from build123d import *

# Parameters (mm, degrees)
F0_W          = 645
F0_H          = 495
F1_DEPTH      = 82
F3_DEPTH      = 322.501
F3_DEPTH_BACK = 495
F5_DEPTH      = 365
F5_DEPTH_BACK = 341
F6_T          = 18
F6_T3_DEPTH   = 505.2074342574
F6_T5_DEPTH   = 651


# Not quite as in the source:
# - a shell that OpenCascade refuses in one call is made with other operations: the cavity is built on its own and cut out


with BuildPart() as f1:
    # F0 (on Top) → F1 (new body)
    with BuildSketch(Plane.XY):
        Rectangle(F0_W, F0_H)
    extrude(amount=-F1_DEPTH)

    # F2 (on Right) → F3 (cut, two sides)
    with BuildSketch(Plane.YZ) as f3_sk:
        Polygon((-277.5, -15), (-277.5, -112), (-217.5, -112), (-234.6037171287, -15), align=None)
        Polygon((277.5, -15), (234.6037171287, -15), (217.5, -112), (277.5, -112), align=None)
    extrude(amount=F3_DEPTH, mode=Mode.SUBTRACT)
    extrude(f3_sk.sketch, amount=-F3_DEPTH_BACK, mode=Mode.SUBTRACT)

    # F4 (on Front) → F5 (cut, two sides)
    with BuildSketch(Plane.XZ) as f5_sk:
        Polygon((-337.5, -15), (-337.5, -185.1384545885), (-277.5, -185.1384545885), (-307.5, -15), align=None)
        Polygon((337.5, -15), (307.5, -15), (277.5415446769, -154.3605614963), (337.5, -156.5929672103), align=None)
    extrude(amount=F5_DEPTH, mode=Mode.SUBTRACT)
    extrude(f5_sk.sketch, amount=-F5_DEPTH_BACK, mode=Mode.SUBTRACT)

    # F6: shell of thickness 18, made by hand


with BuildPart() as f6_core1:
    # F6_t2: copy of F1
    add(f1.part)

    # the walls: a layer under each face that stays
    f6_faces = [f6_core1.faces().sort_by_distance(p)[0] for p in [
        (-322.5, 0, -7.5),
        (0, -247.5, -7.5),
        (322.5, 0, -7.5),
        (314.537037037, -170.15625, -15),
        (0, 228.696763275, -48.5),
        (-1.2945688909, 0, -82),
        (300.2984772553, 0, -48.5),
        (0, -228.696763275, -48.5),
        (-301.5930461463, 0, -48.5),
        (0, 247.5, -7.5),
    ]]
    thicken(f6_faces, amount=-F6_T, mode=Mode.SUBTRACT)

    # F6_s4 → F6_t3 (cut)
    with BuildSketch(Plane.XZ.offset(-252.6037171287)):
        Polygon((-307.6772653955, -15.211256672), (-307.5, 3), (-292.3962066388, 3), (-289.7734604458, -11.874332802), align=None)
        Polygon((307.6759796954, -15.2178305009), (307.5, 3), (292.9582599542, 3), (289.902030457, -11.2169499127), align=None)
    extrude(amount=F6_T3_DEPTH, mode=Mode.SUBTRACT)

    # F6_s6 → F6_t5 (cut)
    with BuildSketch(Plane.YZ.offset(-325.5)):
        Polygon((-234.7809825243, -15.211256672), (-234.6037171287, 3), (-219.4999237675, 3), (-216.8771775745, -11.874332802), align=None)
        Polygon((234.7809825243, -15.211256672), (234.6037171287, 3), (219.4999237675, 3), (216.8771775745, -11.874332802), align=None)
    extrude(amount=F6_T5_DEPTH, mode=Mode.SUBTRACT)


with BuildPart() as f1_1:
    add(f1.part)

    # what is left inside the walls is the cavity
    f6_cavity = [f6_core1.part.solids().sort_by_distance(p)[0] for p in [
        (0.223061, -72.990314, -0.18),
    ]]
    add(f6_cavity, mode=Mode.SUBTRACT)


solid = f1_1.part
Geometry check sheet. Reference: the model listing, model coordinates, mm. A direction names the side the tool comes from. Round coordinates to 2 decimals unless told otherwise and drop trailing zeros. Loops run counter-clockwise (first coordinate to the right, second up) from the corner with the lowest first, then second, coordinate; pieces in that order, holes last.
Item 1: Cross-section at A-A on z = -46. Record the boundary of the cut face in (x, y), then the cut area to 3 significant figures.
Item 2: Cross-section at B-B on y = -13.5. Record the boundary of the cut face in (x, z), then the cut area to 3 significant figures.
Item 3: Gauge pin test, flat ends, axial feed: pin 1 (1.5 mm diameter, centred on y = -141, z = -59, fed in from +X); pin 2 (3 mm diameter, centred on y = 15.5, z = -44, fed in from +X); pin 3 (10 mm diameter, centred on x = -49.5, z = -43.5, fed in from +Y). Record the tip position at first contact, or that the pin passes through.
Item 4: Access from +Z, -Z, +X, -X, +Y, -Y to the whole of each face (thin tool, end or side, straight path). Record for faces 1 (the flat face through (-5, 3, -82)), 2 (the flat face through (285.53, 3.07, -31.55)), 3 (the flat face through (2, 239, -15)).
Item 5: Thickness scan on line 1 (X direction, y = -63.5, z = -12.5); line 2 (X direction, y = 11.5, z = -11.5); line 3 (Y direction, x = 134, z = -27.5). Record the ranges inside material, lowest first.
Item 6: Cross-section at C-C on x = 225. Record the boundary of the cut face in (y, z).
Item 7: Mould release check, pull along X, two halves, no side actions. Record for faces 4 (the flat face through (4.31, 228.78, -48.03)), 5 (the flat face through (-322.5, -3, -7)), 6 (the flat face through (-5, 3, -64)): pulls with the +X half, pulls with the -X half, needs draft (parallel to the pull), parting line crosses it, or undercut.
Answer sheet:
1. outline: (-302.03, -229.14) - (300.84, -229.14) - (300.84, 229.14) - (-302.03, 229.14) - close; hole (-283.76, -210.86) - (282.42, -210.86) - (282.42, 210.86) - (-283.76, 210.86) - close
1. area: 37,500 mm2
2. outline: (-322.5, -15) - (-307.5, -15) - (-295.69, -82) - (293.1, -82) - (307.5, -15) - (322.5, -15) - (322.5, 0) - (292.31, 0) - (278.56, -64) - (-280.58, -64) - (-291.87, 0) - (-322.5, 0) - close
2. area: 13,400 mm2
3. pin 1: stops at x = 298.2
3. pin 2: stops at x = 301.59
3. pin 3: stops at y = 230.46
4. face 1: -Z, +X, -X, +Y, -Y
4. face 2: +Z
4. face 3: -Z
5. line 1: x = -322.5 to -289.66, 289.63 to 322.5
5. line 2: x = -322.5 to -289.84, 289.84 to 322.5
5. line 3: y = -232.4 to -214.12, 214.12 to 232.4
6. outline: (-247.5, -15) - (-234.6, -15) - (-222.79, -82) - (222.79, -82) - (234.6, -15) - (247.5, -15) - (247.5, 0) - (218.97, 0) - (207.69, -64) - (-207.69, -64) - (-218.97, 0) - (-247.5, 0) - close
7. face 4: needs draft
7. face 5: pulls with the -X half
7. face 6: undercut
